Read the model definition and answer for the solid it produces. Units are mm, in the model's axes. Round coordinates to 2 decimals unless told otherwise and drop trailing zeros. Loops run counter-clockwise (first coordinate to the right, second up) from the corner with the lowest first, then second, coordinate; pieces in that order, holes last. Notation, with made-up numbers: M 21.5,66.5 L 58.5,66.5 A17 ccw 58.5,97.5 Z; hole C -3,-37.75 d9. An arc over 180 degrees is marked long. Write each question's results on one line, items separated by ' | '.
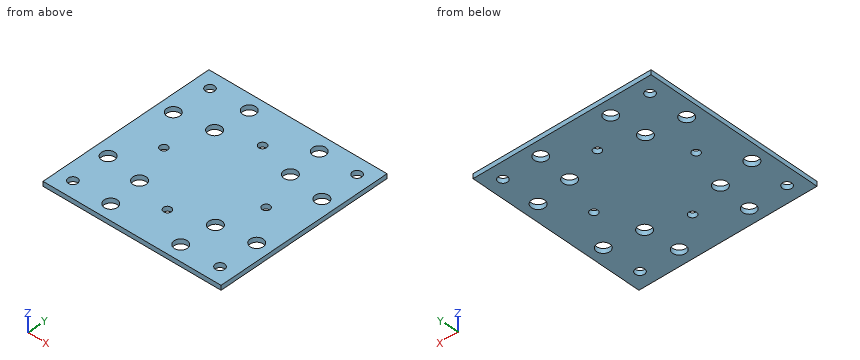
```python
from build123d import *

# Parameters (mm, degrees)
SKETCH_1_W          = 115
SKETCH_1_H          = 115
EXTRUDE_1_DEPTH     = 3
SKETCH_3_R          = 3
CUT_EXTRUDE_2_DEPTH = 82.372599811
SKETCH_4_R          = 4.25
SKETCH_4_R_2        = 2.5
CUT_EXTRUDE_3_DEPTH = 3
SKETCH_5_R          = 4.25
CUT_EXTRUDE_4_DEPTH = 3


with BuildPart() as part:
    # 草图1 → 凸台-拉伸1 (new body)
    with BuildSketch(Plane.XY):
        Rectangle(SKETCH_1_W, SKETCH_1_H)
    extrude(amount=EXTRUDE_1_DEPTH)

    # 草图3 → 切除-拉伸2 (cut, through all)
    with BuildSketch(Plane.XY.offset(3)):
        with Locations((-47.5, 47.5)):
            Circle(SKETCH_3_R)
        with Locations((47.5, 47.5)):
            Circle(SKETCH_3_R)
        with Locations((47.5, -47.5)):
            Circle(SKETCH_3_R)
        with Locations((-47.5, -47.5)):
            Circle(SKETCH_3_R)
    extrude(amount=-CUT_EXTRUDE_2_DEPTH, mode=Mode.SUBTRACT)

    # 草图4 → 切除-拉伸3 (cut)
    with BuildSketch(Plane.XY.offset(3)):
        with Locations((-22.6, -48)):
            Circle(SKETCH_4_R)
        with Locations((22.6, -48)):
            Circle(SKETCH_4_R)
        with Locations((-48, -22.6)):
            Circle(SKETCH_4_R)
        with Locations((-48, 22.6)):
            Circle(SKETCH_4_R)
        with Locations((48, -22.6)):
            Circle(SKETCH_4_R)
        with Locations((48, 22.6)):
            Circle(SKETCH_4_R)
        with Locations((22.6, 48)):
            Circle(SKETCH_4_R)
        with Locations((-22.6, 48)):
            Circle(SKETCH_4_R)
        with Locations((-33, 0)):
            Circle(SKETCH_4_R_2)
        with Locations((0, -33)):
            Circle(SKETCH_4_R_2)
        with Locations((0, 33)):
            Circle(SKETCH_4_R_2)
        with Locations((33, 0)):
            Circle(SKETCH_4_R_2)
    extrude(amount=-CUT_EXTRUDE_3_DEPTH, mode=Mode.SUBTRACT)

    # 草图5 → 切除-拉伸4 (cut)
    with BuildSketch(Plane.XY.offset(3)):
        with Locations((-24.5, 26)):
            Circle(SKETCH_5_R)
        with Locations(Location((-24.5, -26, 0), (0, 0, 180))):
            Circle(SKETCH_5_R)
        with Locations(Location((24.5, 26, 0), (0, 0, 180))):
            Circle(SKETCH_5_R)
        with Locations((24.5, -26)):
            Circle(SKETCH_5_R)
    extrude(amount=-CUT_EXTRUDE_4_DEPTH, mode=Mode.SUBTRACT)


solid = part.part
```
1. Find section B-B, the plane z = 1.65. Count the separate pieces of the cut face and the enclosed holes in it, then the cut area to 3 significant figures.
Completed:
separate pieces: 1 | enclosed holes: 20 | area: 12,400 mm2
2. Find section C-C, the plane x = 24.5. Give the vertices of the cut face in (y, z), then the cut area to 3 significant figures.
Completed:
outline: M -57.5,0 L -51.8,0 L -51.8,3 L -57.5,3 Z; M -44.2,0 L -30.25,0 L -30.25,3 L -44.2,3 Z; M -21.75,0 L 21.75,0 L 21.75,3 L -21.75,3 Z; M 30.25,0 L 44.2,0 L 44.2,3 L 30.25,3 Z; M 51.8,0 L 57.5,0 L 57.5,3 L 51.8,3 Z | area: 248 mm2
3. Find section D-D, the plane x = -48. Give the vertices of the cut face in (y, z), then the cut area to 3 significant figures.
Completed:
outline: M -57.5,0 L -50.46,0 L -50.46,3 L -57.5,3 Z; M -44.54,0 L -26.85,0 L -26.85,3 L -44.54,3 Z; M -18.35,0 L 18.35,0 L 18.35,3 L -18.35,3 Z; M 26.85,0 L 44.54,0 L 44.54,3 L 26.85,3 Z; M 50.46,0 L 57.5,0 L 57.5,3 L 50.46,3 Z | area: 259 mm2
4. Given P1, Ø9.5, axis at x = 47.5, y = 47.5, coming from the -Z side, flat-ended and moving along its own axis, determine where the tip first touches the part or whether it passes through.
Completed:
P1: stops at z = 0
5. Find the intervals of material crossed by L1, parallel to Y at x = 0, z = 2.2; L2, parallel to Y at x = -33, z = 1.35; L3, parallel to Y at x = -47.5, z = 1.35, in increasing order.
Completed:
L1: y = -57.5 to -35.5, -30.5 to 30.5, 35.5 to 57.5 | L2: y = -57.5 to -2.5, 2.5 to 57.5 | L3: y = -57.5 to -50.5, -44.5 to -26.82, -18.38 to 18.38, 26.82 to 44.5, 50.5 to 57.5
6. Find section A-A, the plane x = -33. Give the vertices of the cut face in (y, z).
Completed:
outline: M -57.5,0 L -2.5,0 L -2.5,3 L -57.5,3 Z; M 2.5,0 L 57.5,0 L 57.5,3 L 2.5,3 Z
